The listing builds one solid part. Answer for the finished solid, in the listing's coordinates (mm). A direction names the side the tool comes from. Give positions to 0.01 mm unless a question says otherwise; leave off trailing zeros. Loops run counter-clockwise (first coordinate to the right, second up) from the corner with the lowest first, then second, coordinate; pieces in that order, holes last. Notation, with made-up numbers: M 10.25,-38 L 36.25,-38 A24 cw 36.25,-19 Z; hole C 36,43.5 d6. An arc over 180 degrees is marked long. Use one line per item in the form item = value. Start each with the question number.
1. The part is cut by section D-D (z = 9). Write down the section's boundary in (x, y).
2. Straight lines are drawn through the part: line 1 (Z direction, x = 0, y = -3); line 2 (X direction, y = -2.4, z = 1); line 3 (X direction, y = -0.5, z = 2). For each, find the intervals that lie inside material, in ascending order. Write a range as from..to.
3. The part is cut by section C-C (x = 14.5). Write down the section's boundary in (y, z), and give its area (3 significant figures).
4. The mould has two halves that part along Z. Classify faces 1 (the face through (-2.51, -1.252, -4.267)), 2 (the face through (0, -3.81, -4)), 3 (the face through (16.5, -1.9, 5.2)): released by +Z, released by -Z, zero draft, split by the parting line, or undercut.
5. The part is cut by section B-B (z = 0). Write down the section's boundary in (x, y), and give its area (3 significant figures).
6. Each of these flat-tipped pins is pushed along its axis until it touches: pin 1 Ø1 at (x, y) = (-12, -1) entering from -Z; pin 2 Ø1 at (y, z) = (-1, 6) entering from -X; pin 3 Ø12 at (x, z) = (-7, 10.5) entering from +Y; pin 4 Ø2 at (y, z) = (-1.5, -1.5) entering from -X. Where does it stop, or does it pass through?
7. For faces 4 (the face through (-2.3, -2.54, -2.5)), 5 (the face through (3, -3, 0)), determine the directions among +Z, -Z, +X, -X, +Y, -Y from which every point of the face is accessible in a straight line to the end or side of a thin tool.
8. The part is cut by section A-A (y = -1.1). Write down the section's boundary in (x, z).
from build123d import *

# Parameters (mm, degrees)
F0_R     = 17.299
F1_DEPTH = 3.81
F3_DEPTH = 1.27
F4_DEPTH = 2.54
F5_R     = 3
F6_DEPTH = 3.811


with BuildPart() as f1:
    # F0 (on Front) → F1 (new body)
    with BuildSketch(Plane.XZ):
        Circle(F0_R)
    extrude(amount=F1_DEPTH)

    # F2 (on Front) → F3 (cut)
    with BuildSketch(Plane.XZ):
        Polygon((-4.95, 2.857884), (-4.95, -2.857884), (0, -5.715768), (4.95, -2.857884), (4.95, 2.857884), (0, 5.715768), align=None)
    extrude(amount=F3_DEPTH, mode=Mode.SUBTRACT)

    # F2 (on Front) → F4 (cut)
    with BuildSketch(Plane.XZ):
        Polygon((-4.95, 2.857884), (-4.95, -2.857884), (0, -5.715768), (4.95, -2.857884), (4.95, 2.857884), (0, 5.715768), align=None)
    extrude(amount=F4_DEPTH, mode=Mode.SUBTRACT)

    # F5 (on face) → F6 (cut, through all)
    with BuildSketch(Plane(origin=(0, 0, 0), x_dir=(-1, 0, 0), z_dir=(0, 1, 0))):
        Circle(F5_R)
    extrude(amount=-F6_DEPTH, mode=Mode.SUBTRACT)


solid = f1.part
Derived:
q1.outline = M -14.77,-3.81 L 14.77,-3.81 L 14.77,0 L -14.77,0 Z
q2.line_1 = -17.3..-3, 3..17.3
q2.line_2 = -17.27..-4.95, 4.95..17.27
q2.line_3 = -17.18..-4.95, 4.95..17.18
q3.outline = M -3.81,-9.43 L 0,-9.43 L 0,9.43 L -3.81,9.43 Z
q3.area = 71.9 mm2
q4.face_1 = undercut
q4.face_2 = zero draft
q4.face_3 = split by the parting line
q5.outline = M -17.3,-3.81 L -3,-3.81 L -3,-2.54 L -4.95,-2.54 L -4.95,0 L -17.3,0 Z; M 3,-3.81 L 17.3,-3.81 L 17.3,0 L 4.95,0 L 4.95,-2.54 L 3,-2.54 Z
q5.area = 99.1 mm2
q6.pin_1 = -12.92
q6.pin_2 = -16.4
q6.pin_3 = 0
q6.pin_4 = -17.29
q7.face_4 = +Y
q7.face_5 = +Y, -Y
q8.outline = C 0,0 d34.6; hole M -4.95,-2.86 L 0,-5.72 L 4.95,-2.86 L 4.95,2.86 L 0,5.72 L -4.95,2.86 Z
